Build history of the part. All positions in model axes, mm. Round coordinates to 2 decimals unless told otherwise and drop trailing zeros. Order: outer loops, then holes, each group sorted by start corner. A loop starts at its lowest first (then second) coordinate and runs counter-clockwise, first axis right, second up. Notation, with made-up numbers: (87.25, -4) -> (118.25, -4) arc R30 ccw to (118.25, 26) -> close; hole circle Ø5 at (6.25, 66). An arc over 180 degrees is marked (long way). Use a Markdown table: item, result. Add a question column.
Item 1: Pin check, flat tips, straight feed: pin 1 (5 mm diameter, centred on y = -18, z = -16, fed in from +X); pin 2 (6 mm diameter, centred on y = -18, z = 16, fed in from +X). Stop position of each tip, or through.
Item 2: Slice it at A-A, the plane y = 7.5. Give the cut face in (x, z), plus the area to 3 significant figures.
Item 3: Slice it at B-B, the plane z = -16. State how many separate pieces and enclosed holes the cut face has, plus the area to 3 significant figures.
Item 4: Probe L1, parallel to Z at x = 2.25, y = -18; L2, parallel to Z at x = 2.95, y = 7.5; L3, parallel to Y at x = 2, z = -15. List the from-to ranges inside material, lowest first.
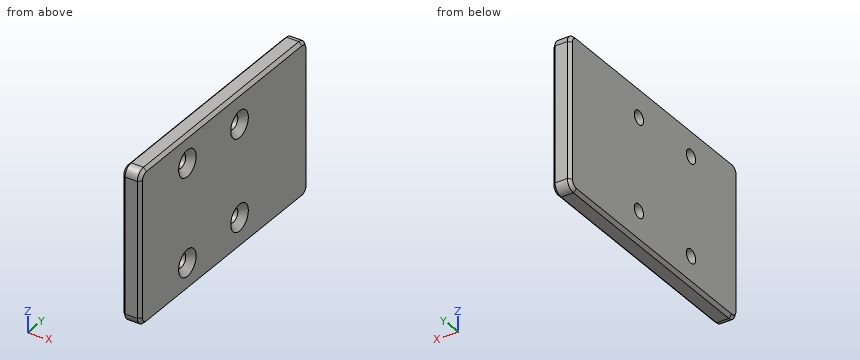
from build123d import *

# Parameters (mm, degrees)
SKETCH_1_W                   = 50
SKETCH_1_H                   = 82
EXTRUDE_1_DEPTH              = 6
FILLET_1_R                   = 3
CHAMFER_1_SIZE               = 1
HOLE_WIZARD_M4_1_D           = 4.5
HOLE_WIZARD_M4_1_CSINK_D     = 8.6
HOLE_WIZARD_M4_1_CSINK_ANGLE = 90


with BuildPart() as part:
    # 草图1 → 凸台-拉伸1 (new body)
    with BuildSketch(Plane(origin=(0, 0, 0), x_dir=(0, 0, -1), z_dir=(1, 0, 0))):
        Rectangle(SKETCH_1_W, SKETCH_1_H)
    extrude(amount=EXTRUDE_1_DEPTH)

    # 圆角1
    fillet_1_edges = [part.edges().sort_by_distance(p)[0] for p in [
        (3, -41, -25),
        (3, -41, 25),
        (3, 41, 25),
        (3, 41, -25),
    ]]
    fillet(fillet_1_edges, radius=FILLET_1_R)

    # 倒角1
    chamfer_1_edges = [part.edges().sort_by_distance(p)[0] for p in [
        (0, -41, 0),
        (6, -41, 0),
        (0, 0, -25),
        (0, 0, 25),
        (0, 41, 0),
        (0, 40.121320344, -24.121320344),
        (0, 40.121320344, 24.121320344),
        (0, -40.121320344, -24.121320344),
        (0, -40.121320344, 24.121320344),
        (6, 0, 25),
        (6, 0, -25),
        (6, 41, 0),
        (6, 40.121320344, -24.121320344),
        (6, 40.121320344, 24.121320344),
        (6, -40.121320344, -24.121320344),
        (6, -40.121320344, 24.121320344),
    ]]
    chamfer(chamfer_1_edges, length=CHAMFER_1_SIZE)

    # M4 十字槽沉头木螺钉的锥形沉头孔1 (through all)
    with Locations(Plane(origin=(6, 0, 0), x_dir=(0, 0, -1), z_dir=(1, 0, 0))):
        with Locations((15, 7.5), (-15, 7.5), (16, -18), (-16, -18)):
            CounterSinkHole(HOLE_WIZARD_M4_1_D / 2, HOLE_WIZARD_M4_1_CSINK_D / 2, counter_sink_angle=HOLE_WIZARD_M4_1_CSINK_ANGLE)


solid = part.part
Check sheet entries:
| question | item | result |
|---|---|---|
| 1 | pin 1 | x = 4.2 |
| 1 | pin 2 | x = 4.7 |
| 2 | outline | (0, -24) -> (1, -25) -> (5, -25) -> (6, -24) -> (6, -19.3) -> (3.95, -17.25) -> (0, -17.25) -> close; (0, -12.75) -> (3.95, -12.75) -> (6, -10.7) -> (6, 10.7) -> (3.95, 12.75) -> (0, 12.75) -> close; (0, 17.25) -> (3.95, 17.25) -> (6, 19.3) -> (6, 24) -> (5, 25) -> (1, 25) -> (0, 24) -> close |
| 2 | area | 236 mm2 |
| 3 | separate pieces | 3 |
| 3 | enclosed holes | 0 |
| 3 | area | 430 mm2 |
| 4 | L1 | -25 to -18.25, -13.75 to 13.75, 18.25 to 25 |
| 4 | L2 | -25 to -17.25, -12.75 to 12.75, 17.25 to 25 |
| 4 | L3 | -41 to -20.02, -15.98 to 5.25, 9.75 to 41 |
